Geometry: final body of the model. Coordinates: model frame, mm. Round coordinates to 2 decimals unless told otherwise and drop trailing zeros. Use one line per item in the form item = value. Start each with the question number.
1. Draft query along X for faces 1 (the face through (-2.09, -0.02, -3.556)), 2 (the face through (2.03, -0.02, -3.59)), 3 (the face through (0, -1.588, -2)), 4 (the face through (-0.34, -0.02, -1.55)). Return one class per face: pulls with the +X half, pulls with the -X half, needs draft (parallel to the pull), parting line crosses it, or undercut.
2. Pin query (flat end, axial travel): pin 1 Ø1 at (x, y) = (-1.5, 1) entering from -Z. Return the tip coordinate at first contact, or that it passes through.
3. Line query: L1, parallel to Z at x = 0, y = 0.1; L2, parallel to Z at x = 0.5, y = 0.5; L3, parallel to X at y = -1.3, z = 1. Output: solid intervals per line, ascending.
```python
from build123d import *

# Parameters (mm, degrees)
F1_DEPTH = 1.5875
F2_R     = 1.5875
F3_DEPTH = 3.176
F4_R     = 0.127
F5_R     = 0.254


with BuildPart() as f1:
    # F0 (on Front) → F1 (new body, symmetric)
    with BuildSketch(Plane.XZ):
        Polygon((4.1245009758, 2.3811547516), (0.0001099827, 4.7624999987), (-4.1243909931, 2.3813452472), (-4.1245009758, -2.3811547516), (-0.0001099827, -4.7624999987), (4.1243909931, -2.3813452472), align=None)
    extrude(amount=F1_DEPTH, both=True)

    # F2 (on face) → F3 (cut, through all)
    with BuildSketch(Plane.XZ.offset(1.5875)):
        Circle(F2_R)
    extrude(amount=-F3_DEPTH, mode=Mode.SUBTRACT)

    # F4
    f4_edges = [f1.edges().sort_by_distance(p)[0] for p in [
        (-2.062141, -1.5875, 3.571923),
        (-4.124446, -1.5875, 9.5e-05),
        (2.062305, -1.5875, 3.571827),
        (-2.062305, -1.5875, -3.571827),
        (2.062141, -1.5875, -3.571923),
        (4.124446, -1.5875, -9.5e-05),
        (4.124501, 0, 2.381155),
        (0.00011, 0, 4.7625),
        (4.124446, 1.5875, -9.5e-05),
        (2.062305, 1.5875, 3.571827),
        (-4.124446, 1.5875, 9.5e-05),
        (-2.062141, 1.5875, 3.571923),
        (2.062141, 1.5875, -3.571923),
        (4.124391, 0, -2.381345),
        (-2.062305, 1.5875, -3.571827),
        (-0.00011, 0, -4.7625),
        (-4.124501, 0, -2.381155),
        (-4.124391, 0, 2.381345),
    ]]
    fillet(f4_edges, radius=F4_R)

    # F5
    f5_edges = [f1.edges().sort_by_distance(p)[0] for p in [
        (-1.998643, -1.5875, 3.461936),
        (1.998803, -1.5875, 3.461844),
        (-3.997446, -1.5875, 9.2e-05),
        (3.997446, -1.5875, -9.2e-05),
        (-1.998803, -1.5875, -3.461844),
        (1.998643, -1.5875, -3.461936),
        (-1.5875, -1.5875, 0),
        (1.5875, 0, 0),
        (-1.5875, 1.5875, 0),
    ]]
    fillet(f5_edges, radius=F5_R)


solid = f1.part
```
Outcome:
q1.face_1 = pulls with the -X half
q1.face_2 = pulls with the +X half
q1.face_3 = needs draft
q1.face_4 = undercut
q2.pin_1 = -4.19
q3.L1 = -4.74 to -1.59, 1.59 to 4.74
q3.L2 = -4.47 to -1.51, 1.51 to 4.47
q3.L3 = -4.12 to -1.23, 1.23 to 4.12
